Verification items for the finished model (mm, model axes). Face numbers are marked on the shaded views. A direction names the side the tool comes from. Give positions to 0.01 mm unless a question says otherwise; leave off trailing zeros. Loops run counter-clockwise (first coordinate to the right, second up) from the corner with the lowest first, then second, coordinate; pieces in that order, holes last. Notation, with made-up numbers: (47.5, 6.5) - (103.5, 6.5) arc R33 cw to (103.5, 36.5) - close; hole circle Ø4 at (56.5, -9.75). An arc over 180 degrees is marked (long way). One line per question, with ' | ' between items. Start each with the question number.
1. Tool access check on the marked faces 1, 2 and 3. Record the directions out of +Z, -Z, +X, -X, +Y, -Y that give a thin tool (end or side, any length) a straight path to the whole face; none if there is none.
2. Mould release check, pull along Z, two halves, no side actions. Record for the marked faces 4, 5 and 6: +Z half, -Z half, draft (parallel to the pull), parting line (faces both ways), or undercut.
3. Thickness scan on line 1 along Z through (x, y) = (85.5, 40.5); line 2 along Y through (x, z) = (-0.5, 256.5). Record the ranges inside material, lowest first. Write a range as from..to.
4. Section check C-C, the plane z = 197. Enter the section's corners in (x, y), then the cut area to 3 significant figures.
5. Depth check by flat-ended pin: pin 1 Ø6 at (x, y) = (250.5, -121.5) entering from -Z. Enter the tip coordinate at first touch or a pass-through.
6. Section check A-A, the plane y = 85.5. Enter the section's corners in (x, z).
7. Section check B-B, the plane x = 86. Enter the section's corners in (y, z).
8. Section check D-D, the plane x = 391.5. Enter the section's corners in (y, z).
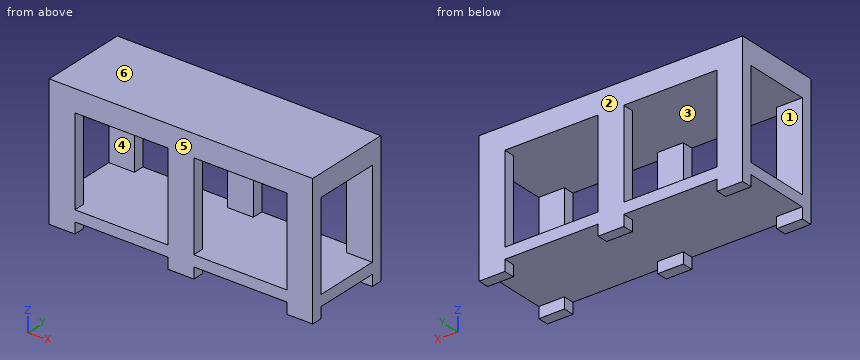
from build123d import *

# Parameters (mm, degrees)
F0_W     = 914.4
F0_H     = 304.8
F1_DEPTH = 457.2
F2_W     = 323.85
F2_H     = 304.8
F3_DEPTH = 304.801
F4_W     = 228.6
F4_H     = 304.8
F5_DEPTH = 914.401
F6_W     = 323.85
F6_H     = 38.1
F7_DEPTH = 304.801
F8_W     = 228.6
F8_H     = 38.1
F9_DEPTH = 914.401


with BuildPart() as f1:
    # F0 (on Top) → F1 (new body)
    with BuildSketch(Plane.XY):
        Rectangle(F0_W, F0_H)
    extrude(amount=F1_DEPTH)

    # F2 (on face) → F3 (cut, through all)
    with BuildSketch(Plane.XZ.offset(152.4)):
        with Locations((-206.375, 228.6)):
            Rectangle(F2_W, F2_H)
        with Locations((206.375, 228.6)):
            Rectangle(F2_W, F2_H)
    extrude(amount=-F3_DEPTH, mode=Mode.SUBTRACT)

    # F4 (on face) → F5 (cut, through all)
    with BuildSketch(Plane.YZ.offset(457.2)):
        with Locations((0, 228.6)):
            Rectangle(F4_W, F4_H)
    extrude(amount=-F5_DEPTH, mode=Mode.SUBTRACT)

    # F6 (on face) → F7 (cut, through all)
    with BuildSketch(Plane.XZ.offset(152.4)):
        with Locations((-206.375, 19.05)):
            Rectangle(F6_W, F6_H)
        with Locations((206.375, 19.05)):
            Rectangle(F6_W, F6_H)
    extrude(amount=-F7_DEPTH, mode=Mode.SUBTRACT)

    # F8 (on face) → F9 (cut, through all)
    with BuildSketch(Plane.YZ.offset(457.2)):
        with Locations((0, 19.05)):
            Rectangle(F8_W, F8_H)
    extrude(amount=-F9_DEPTH, mode=Mode.SUBTRACT)


solid = f1.part
Results list:
1) face 1: +X, -X | face 2: +Z, -Z, +X, -X, +Y | face 3: none
2) face 4: undercut | face 5: draft | face 6: +Z half
3) line 1: 38.1..76.2, 381..457.2 | line 2: -152.4..-114.3, 114.3..152.4
4) outline: (-457.2, -152.4) - (-368.3, -152.4) - (-368.3, -114.3) - (-457.2, -114.3) - close; (-457.2, 114.3) - (-368.3, 114.3) - (-368.3, 152.4) - (-457.2, 152.4) - close; (-44.45, -152.4) - (44.45, -152.4) - (44.45, -114.3) - (-44.45, -114.3) - close; (-44.45, 114.3) - (44.45, 114.3) - (44.45, 152.4) - (-44.45, 152.4) - close; (368.3, -152.4) - (457.2, -152.4) - (457.2, -114.3) - (368.3, -114.3) - close; (368.3, 114.3) - (457.2, 114.3) - (457.2, 152.4) - (368.3, 152.4) - close | area: 20,300 mm²
5) pin 1: z = 38.1
6) outline: (-457.2, 38.1) - (457.2, 38.1) - (457.2, 76.2) - (-457.2, 76.2) - close; (-457.2, 381) - (457.2, 381) - (457.2, 457.2) - (-457.2, 457.2) - close
7) outline: (-152.4, 38.1) - (152.4, 38.1) - (152.4, 76.2) - (-152.4, 76.2) - close; (-152.4, 381) - (152.4, 381) - (152.4, 457.2) - (-152.4, 457.2) - close
8) outline: (-152.4, 0) - (-114.3, 0) - (-114.3, 38.1) - (114.3, 38.1) - (114.3, 0) - (152.4, 0) - (152.4, 457.2) - (-152.4, 457.2) - close; hole (-114.3, 76.2) - (114.3, 76.2) - (114.3, 381) - (-114.3, 381) - close
